Can you work these out from the model? Positions are in its coordinate system, mm. A direction names the side the tool comes from. Give positions to 0.01 mm unless a question says otherwise; leave off trailing zeros. Loops run counter-clockwise (first coordinate to the right, second up) from the corner with the lowest first, then second, coordinate; pieces in that order, holes last. Notation, with made-up numbers: (-0.5, -35) -> (34.5, -35) arc R15 ccw to (34.5, -26) -> close; hole circle Ø7 at (88.25, 6.5). An arc over 180 degrees is marked (long way). One line per question, with ' | ' between items.
Autodesk Inventor part; units mm, degrees
ref_plane "YZ Plane" through (0, 0, 0) normal (1, 0, 0) x (0, 1, 0)
ref_plane "XZ Plane" through (0, 0, 0) normal (0, 1, 0) x (-1, 0, 0)
ref_plane "XY Plane" through (0, 0, 0) normal (0, 0, 1) x (1, 0, 0)
sketch "Sketch15" plane through (0, 0, 0) normal (1, 0, 0) x (0, 1, 0)
  line L0 (0, 0) -> (50.8, 0)
  line L1 (50.8, 0) -> (50.8, 25.4)
  line L2 (50.8, 25.4) -> (0, 25.4)
  line L3 (0, 25.4) -> (0, 0)
  line L4 (48.26, 22.86) -> (2.54, 22.86)
  line L5 (2.54, 22.86) -> (2.54, 2.54)
  line L6 (2.54, 2.54) -> (48.26, 2.54)
  line L7 (48.26, 2.54) -> (48.26, 22.86)
  dimension "d46" = 25.4
  dimension "d47" = 50.8
  dimension "d48" = 2.54
  dimension "d49" = 2.54
  dimension "d50" = 2.54
  dimension "d51" = 2.54
extrude "Extrusion12" add sketch "Sketch15" along normal blind 76.2
sketch "Sketch16" plane through (0, 0, 0) normal (0, 0, -1) x (-1, 0, 0)
  line L0 (0, 0) -> (-76.2, 0)
  line L1 (-76.2, 0) -> (-101.6, 0)
  line L2 (-101.6, 0) -> (-101.6, 50.8)
  line L3 (-101.6, 50.8) -> (-76.2, 50.8)
  line L4 (-76.2, 50.8) -> (-76.2, 0)
  line L5 (-78.74, 48.26) -> (-99.06, 48.26)
  line L6 (-99.06, 48.26) -> (-99.06, 2.54)
  line L7 (-99.06, 2.54) -> (-78.74, 2.54)
  line L8 (-78.74, 2.54) -> (-78.74, 48.26)
  dimension "d54" = 25.4
  dimension "d55" = 50.8
  dimension "d56" = 2.54
  dimension "d57" = 2.54
  dimension "d58" = 2.54
  dimension "d59" = 2.54
extrude "Extrusion13" add sketch "Sketch16" against normal blind 254
sketch "Sketch17" plane through (0, 0, 0) normal (0, 0, -1) x (-1, 0, 0)
  line L0 (0, 2.54) -> (-76.2, 2.54)
  line L1 (0, 48.26) -> (-76.2, 48.26)
  line L2 (-73.617, 2.54) -> (-3.1161, 2.54)
  line L3 (-3.1161, 2.54) -> (-3.1161, 48.26)
  line L4 (-3.1161, 48.26) -> (-73.617, 48.26)
  line L5 (-73.617, 48.26) -> (-73.617, 2.54)
  point P0 (0, 0)
extrude "Extrusion14" add sketch "Sketch17" along normal blind 2.54
equation "\"d49\" = d48"
equation "\"d50\" = d48"
equation "\"d51\" = d48"
equation "\"d56\" = d48"
equation "\"d57\" = d48"
equation "\"d58\" = d48"
equation "\"d59\" = d48"
properties part number "right arm"
Q1. For pin 1 Ø5 at (y, z) = (32, 57.5) entering from -X; pin 2 Ø0.8 at (y, z) = (19, -1.5) entering from -X; pin 3 Ø1.3 at (y, z) = (33.5, -2) entering from +X, each with a flat end and sliding along its axis, tell me the tip position at first contact or that it passes through.
Entries:
pin 1: x = 76.2 | pin 2: x = 3.12 | pin 3: x = 73.62
Q2. If we section it at A-A (z = 145): Write out the boundary of the cut face in (x, y), plus the area to 3 significant figures.
Entries:
outline: (76.2, 0) -> (101.6, 0) -> (101.6, 50.8) -> (76.2, 50.8) -> close; hole (78.74, 2.54) -> (99.06, 2.54) -> (99.06, 48.26) -> (78.74, 48.26) -> close | area: 361 mm²
Q3. If we mould it in two halves opening along Z, with no side actions, what happens to faces 1 (the face through (38, 26, 22.86)), 2 (the face through (0, 23, 2)), 3 (the face through (38, 26, 25.4))? For each: pulls with the +Z half, pulls with the -Z half, needs draft (parallel to the pull), parting line crosses it, or undercut.
Entries:
face 1: undercut | face 2: needs draft | face 3: pulls with the +Z half
Q4. On a 3-axis mill with a long thin cutter (end or side, diameter ignored), from which of +Z, -Z, +X, -X, +Y, -Y can I reach the whole of each face in a straight line? I mean faces 4 (the face through (78.74, 25, 125)), 5 (the face through (39, 26, -2.54)), 6 (the face through (99.3, 27.4, 254)), 7 (the face through (38, 2.54, 13)), 8 (the face through (76.2, 26, 138)). Say none if no direction works.
Entries:
face 4: +Z, -Z | face 5: -Z, +X, -X, +Y, -Y | face 6: +Z, +X, -X, +Y, -Y | face 7: -X | face 8: +Z, -X, +Y, -Y
Q5. If we section it at B-B (y = 10.5): Write out the boundary of the cut face in (x, z), plus the area to 3 significant figures.
Entries:
outline: (0, 0) -> (3.12, 0) -> (3.12, -2.54) -> (73.62, -2.54) -> (73.62, 0) -> (78.74, 0) -> (78.74, 254) -> (76.2, 254) -> (76.2, 25.4) -> (0, 25.4) -> (0, 22.86) -> (76.2, 22.86) -> (76.2, 2.54) -> (0, 2.54) -> close; (99.06, 0) -> (101.6, 0) -> (101.6, 254) -> (99.06, 254) -> close | area: 1,860 mm²
Q6. If we section it at C-C (x = 42): Write out the boundary of the cut face in (y, z).
Entries:
outline: (0, 0) -> (2.54, 0) -> (2.54, -2.54) -> (48.26, -2.54) -> (48.26, 0) -> (50.8, 0) -> (50.8, 25.4) -> (0, 25.4) -> close; hole (2.54, 2.54) -> (48.26, 2.54) -> (48.26, 22.86) -> (2.54, 22.86) -> close
Q7. If I drill on probe 1 along X at (y, z) = (3.5, 218.5); probe 2 along Z at (x, y) = (39, 40); probe 3 along X at (y, z) = (2, 125.5), over which ranges is the centre line in solid material (lowest first)? Write a range as from..to.
Entries:
probe 1: 76.2..78.74, 99.06..101.6 | probe 2: -2.54..2.54, 22.86..25.4 | probe 3: 76.2..101.6
